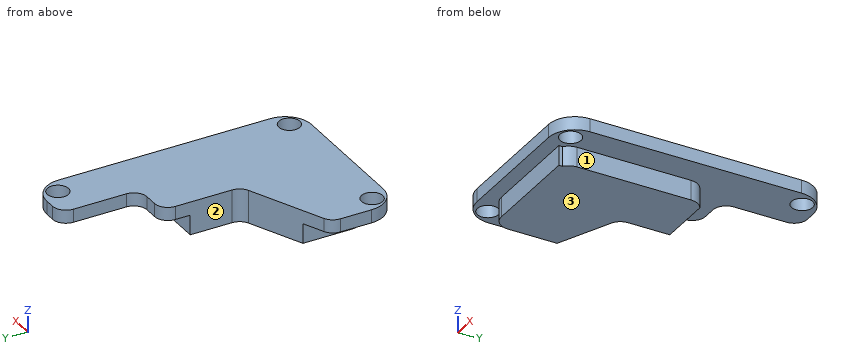
Autodesk Inventor part; units mm, degrees
ref_plane "YZ Plane" through (0, 0, 0) normal (1, 0, 0) x (0, 1, 0)
ref_plane "XZ Plane" through (0, 0, 0) normal (0, 1, 0) x (-1, 0, 0)
ref_plane "XY Plane" through (0, 0, 0) normal (0, 0, 1) x (1, 0, 0)
ref_plane "Arbeitsebene1" through (0, 0, 0) normal (0, 0, 1) x (1, 0, 0)
sketch "Skizze1" plane through (0, 0, 0) normal (0, 0, 1) x (1, 0, 0)
  line L0 (31.9586, -24.4) -> (31.9586, -21.8494)
  line L1 (31.9586, -24.4) -> (35.5793, -24.4)
  arc A0 (35.5793, -24.4) -> (36.5793, -23.4) centre (35.5793, -23.4) ccw
  line L2 (36.5793, -23.4) -> (36.5793, 14.6)
  arc A1 (36.5793, 14.6) -> (35.5793, 15.6) centre (35.5793, 14.6) ccw
  line L3 (35.5793, 15.6) -> (31.5586, 15.6)
  line L4 (31.5586, 15.6) -> (31.5586, -0.3724)
  arc A2 (32.766, -2.6793) -> (31.5586, -0.3724) centre (29.9586, -2.6793) ccw
  line L5 (32.766, -2.6793) -> (32.766, -19.8793)
  arc A3 (31.9586, -21.8494) -> (32.766, -19.8793) centre (29.9586, -19.8793) ccw
  line L6 (20.9586, -22.6867) -> (20.9586, -24.4)
  line L7 (20.9586, -22.6867) -> (16.1586, -22.6867)
  arc A4 (13.3512, -19.8793) -> (16.1586, -22.6867) centre (16.1586, -19.8793) ccw
  line L8 (13.3512, -19.8793) -> (13.3512, -2.6793)
  arc A5 (14.5586, -0.3724) -> (13.3512, -2.6793) centre (16.1586, -2.6793) ccw
  line L9 (14.5586, -0.3724) -> (14.5586, 15.6)
  line L10 (14.5586, 15.6) -> (10.5793, 15.6)
  arc A6 (10.5793, 15.6) -> (9.5793, 14.6) centre (10.5793, 14.6) ccw
  line L11 (9.5793, 14.6) -> (9.5793, -23.4)
  arc A7 (9.5793, -23.4) -> (10.5793, -24.4) centre (10.5793, -23.4) ccw
  line L12 (10.5793, -24.4) -> (20.9586, -24.4)
  circle A8 centre (12.0668, 4.4966) radius 1.4
  line L13 (31.5586, 15.6) -> (14.5586, 15.6)
  line L14 (31.9586, -24.4) -> (20.9586, -24.4)
  line L15 (10.5793, 15.6) -> (9.5793, 15.6)
  line L16 (9.5793, 15.6) -> (9.5793, 14.6)
  line L17 (35.5793, 15.6) -> (36.5793, 15.6)
  line L18 (36.5793, 15.6) -> (36.5793, 14.6)
  line L19 (9.5793, -23.4) -> (9.5793, -24.4)
  line L20 (9.5793, -24.4) -> (10.5793, -24.4)
  line L21 (35.5793, -24.4) -> (36.5793, -24.4)
  line L22 (36.5793, -24.4) -> (36.5793, -23.4)
extrude "Extrusion1" add sketch "Skizze1" along normal blind 2 contours L14 L6 L7 A4 L8 A5 L9 L13 L4 A2 L5 A3 L0 | L0 A3 L5 A2 L4 L3 A1 L2 A0 L1 | A0 L22 L21 | L12 A7 L11 A6 L10 L9 A5 L8 A4 L7 L6 | L20 L19 A7 | A1 L17 L18 | L16 L15 A6 | A8
ref_plane "Arbeitsebene2" through (0, 0, 0) normal (0, 0, 1) x (1, 0, 0)
sketch "Skizze2" plane through (0, 0, 2) normal (0, 0, 1) x (1, 0, 0)
  arc A0 (35.5793, -24.4) -> (36.5793, -23.4) centre (35.5793, -23.4) ccw
  line L0 (36.5793, -23.4) -> (36.5793, 14.6)
  arc A1 (36.5793, 14.6) -> (35.5793, 15.6) centre (35.5793, 14.6) ccw
  line L1 (35.5793, 15.6) -> (10.5793, 15.6)
  arc A2 (10.5793, 15.6) -> (9.5793, 14.6) centre (10.5793, 14.6) ccw
  line L2 (9.5793, 14.6) -> (9.5793, -23.4)
  arc A3 (9.5793, -23.4) -> (10.5793, -24.4) centre (10.5793, -23.4) ccw
  line L3 (10.5793, -24.4) -> (35.5793, -24.4)
  line L4 (34.0793, 13.1) -> (34.0793, -21.9)
  line L5 (34.0793, -21.9) -> (12.0793, -21.9)
  line L6 (12.0793, -21.9) -> (12.0793, 13.1)
  line L7 (12.0793, 13.1) -> (34.0793, 13.1)
  point P0 (8.0712, 15)
  point P1 (8.0712, -15)
  point P2 (38.0712, 15)
  point P3 (38.0712, -15)
  dimension "d21" = 2.5
hole "Bohrung1" at (34.0793, 13.1, 2) at (34.0793, -21.9, 2) at (12.0793, -21.9, 2) at (12.0793, 13.1, 2) direction (0, 0, -1) diameter 3.2 end through all
sketch "Skizze4" plane through (0, 0, 0) normal (0, 0, -1) x (-1, 0, 0)
  circle A0 centre (-34.0793, 13.1) radius 1.4
  circle A1 centre (-34.0793, -21.9) radius 1.4
  line L0 (-31.9586, -24.4) -> (-31.9586, -21.8494)
  line L1 (-31.9586, -24.4) -> (-35.5793, -24.4)
  arc A2 (-36.5793, -23.4) -> (-35.5793, -24.4) centre (-35.5793, -23.4) ccw
  line L2 (-36.5793, -23.4) -> (-36.5793, 14.6)
  arc A3 (-35.5793, 15.6) -> (-36.5793, 14.6) centre (-35.5793, 14.6) ccw
  line L3 (-35.5793, 15.6) -> (-31.5586, 15.6)
  line L4 (-31.5586, 15.6) -> (-31.5586, -0.3724)
  arc A4 (-31.5586, -0.3724) -> (-32.766, -2.6793) centre (-29.9586, -2.6793) ccw
  line L5 (-32.766, -2.6793) -> (-32.766, -19.8793)
  arc A5 (-32.766, -19.8793) -> (-31.9586, -21.8494) centre (-29.9586, -19.8793) ccw
  circle A6 centre (-12.0793, -21.9) radius 1.4
  circle A7 centre (-12.0793, 13.1) radius 1.4
  line L6 (-20.9586, -22.6867) -> (-20.9586, -24.4)
  line L7 (-20.9586, -22.6867) -> (-16.1586, -22.6867)
  arc A8 (-16.1586, -22.6867) -> (-13.3512, -19.8793) centre (-16.1586, -19.8793) ccw
  line L8 (-13.3512, -19.8793) -> (-13.3512, -2.6793)
  arc A9 (-13.3512, -2.6793) -> (-14.5586, -0.3724) centre (-16.1586, -2.6793) ccw
  line L9 (-14.5586, -0.3724) -> (-14.5586, 15.6)
  line L10 (-14.5586, 15.6) -> (-10.5793, 15.6)
  arc A10 (-9.5793, 14.6) -> (-10.5793, 15.6) centre (-10.5793, 14.6) ccw
  line L11 (-9.5793, 14.6) -> (-9.5793, -23.4)
  arc A11 (-10.5793, -24.4) -> (-9.5793, -23.4) centre (-10.5793, -23.4) ccw
  line L12 (-10.5793, -24.4) -> (-20.9586, -24.4)
  circle A12 centre (-12.0668, 4.4966) radius 1.4
  line L13 (-31.0586, -0.651) -> (-31.0586, 16.1)
  line L14 (-31.0586, 16.1) -> (-35.5793, 16.1)
  arc A13 (-35.5793, 16.1) -> (-37.0793, 14.6) centre (-35.5793, 14.6) ccw
  line L15 (-37.0793, 14.6) -> (-37.0793, -23.4)
  arc A14 (-37.0793, -23.4) -> (-35.5793, -24.9) centre (-35.5793, -23.4) ccw
  line L16 (-35.5793, -24.9) -> (-31.4586, -24.9)
  line L17 (-31.4586, -24.9) -> (-31.4586, -21.6326)
  arc A15 (-32.266, -19.8793) -> (-31.4586, -21.6326) centre (-29.9586, -19.8793) ccw
  line L18 (-32.266, -19.8793) -> (-32.266, -2.6793)
  arc A16 (-31.0586, -0.651) -> (-32.266, -2.6793) centre (-29.9586, -2.6793) ccw
  line L19 (-15.0586, 16.1) -> (-15.0586, -0.651)
  arc A17 (-13.8512, -2.6793) -> (-15.0586, -0.651) centre (-16.1586, -2.6793) ccw
  line L20 (-13.8512, -2.6793) -> (-13.8512, -19.8793)
  arc A18 (-16.1586, -22.1867) -> (-13.8512, -19.8793) centre (-16.1586, -19.8793) ccw
  line L21 (-16.1586, -22.1867) -> (-21.4586, -22.1867)
  line L22 (-21.4586, -24.4607) -> (-21.4586, -24.9)
  line L23 (-21.4586, -24.9) -> (-10.5793, -24.9)
  arc A19 (-10.5793, -24.9) -> (-9.0793, -23.4) centre (-10.5793, -23.4) ccw
  line L24 (-9.0793, -23.4) -> (-9.0793, 14.6)
  arc A20 (-9.0793, 14.6) -> (-10.5793, 16.1) centre (-10.5793, 14.6) ccw
  line L25 (-10.5793, 16.1) -> (-15.0586, 16.1)
  line L26 (-31.0586, 15.6607) -> (-15.0586, 15.6607)
  line L27 (-31.4586, -24.4607) -> (-21.4586, -24.4607)
  line L28 (-15.0586, -0.651) -> (-31.0586, -0.651)
  line L29 (-20.9586, -22.6867) -> (-20.9586, -22.1867)
  line L30 (-20.9586, -22.1867) -> (-31.9586, -22.1867)
  point P0 (0, 0)
  point P1 (-31.4586, -22.1867)
  dimension "d22" = 0.5
  dimension "d23" = 0.5
extrude "Extrusion2" add sketch "Skizze4" along normal blind 3 contours L28 A17 L20 A18 L21 L30 L17 A15 L18 A16
fillet "Rundung2" radius 4 4 edges at (9.5793, 15.6, 1) (36.5793, 15.6, 1) (9.5793, -24.4, 1) (36.5793, -24.4, 1)
sketch "Skizze5" plane through (0, 0, 0) normal (0, 0, -1) x (-1, 0, 0)
  circle A0 centre (-23.0793, -4.4) radius 4.25
  circle A1 centre (-12.0668, 4.4966) radius 1.4
  circle A2 centre (-34.0668, 4.4966) radius 1.4
  circle A3 centre (-12.0793, 13.1) radius 1.4
  circle A4 centre (-34.0793, -21.9) radius 1.4
  circle A5 centre (-34.0793, 13.1) radius 1.4
  circle A6 centre (-12.0793, -21.9) radius 1.4
  arc A7 (-29.0793, 13.6) -> (-31.0793, 15.6) centre (-31.0793, 13.6) ccw
  line L0 (-32.5793, 15.6) -> (-31.0793, 15.6)
  arc A8 (-32.5793, 15.6) -> (-36.5793, 11.6) centre (-32.5793, 11.6) ccw
  line L1 (-36.5793, -20.4) -> (-36.5793, 11.6)
  arc A9 (-36.5793, -20.4) -> (-32.5793, -24.4) centre (-32.5793, -20.4) ccw
  line L2 (-13.5793, -24.4) -> (-32.5793, -24.4)
  arc A10 (-13.5793, -24.4) -> (-9.5793, -20.4) centre (-13.5793, -20.4) ccw
  line L3 (-9.5793, 11.6) -> (-9.5793, -20.4)
  arc A11 (-9.5793, 11.6) -> (-13.5793, 15.6) centre (-13.5793, 11.6) ccw
  line L4 (-15.0793, 15.6) -> (-13.5793, 15.6)
  arc A12 (-15.0793, 15.6) -> (-17.0793, 13.6) centre (-15.0793, 13.6) ccw
  line L5 (-17.0793, 13.6) -> (-17.0793, 5.6)
  arc A13 (-19.0793, 3.6) -> (-17.0793, 5.6) centre (-19.0793, 5.6) ccw
  line L6 (-19.0793, 3.6) -> (-27.0793, 3.6)
  arc A14 (-29.0793, 5.6) -> (-27.0793, 3.6) centre (-27.0793, 5.6) ccw
  line L7 (-29.0793, 5.6) -> (-29.0793, 13.6)
  line L8 (-32.5793, 15.6) -> (-13.5793, 15.6)
  point P0 (0, 0)
extrude "Extrusion3" cut sketch "Skizze5" against normal blind 10 contours A7 L8 A12 L5 A13 L6 A14 L7
sketch "Skizze6" plane through (0, 0, 2) normal (0, 0, 1) x (1, 0, 0)
  line L0 (19.0793, 3.6) -> (27.0793, 3.6)
  line L1 (23.0793, 3.6) -> (23.0793, -8.2849)
  line L2 (23.0793, -8.2849) -> (9.5499, -14.3825)
  circle A0 centre (12.0793, 13.1) radius 1.6
  circle A1 centre (34.0793, -21.9) radius 1.6
  circle A2 centre (34.0793, 13.1) radius 1.6
  circle A3 centre (12.0793, -21.9) radius 1.6
  arc A4 (31.0793, 15.6) -> (29.0793, 13.6) centre (31.0793, 13.6) ccw
  line L3 (29.0793, 13.6) -> (29.0793, 5.6)
  arc A5 (27.0793, 3.6) -> (29.0793, 5.6) centre (27.0793, 5.6) ccw
  line L4 (27.0793, 3.6) -> (19.0793, 3.6)
  arc A6 (17.0793, 5.6) -> (19.0793, 3.6) centre (19.0793, 5.6) ccw
  line L5 (17.0793, 5.6) -> (17.0793, 13.6)
  arc A7 (17.0793, 13.6) -> (15.0793, 15.6) centre (15.0793, 13.6) ccw
  line L6 (15.0793, 15.6) -> (13.5793, 15.6)
  arc A8 (13.5793, 15.6) -> (9.5793, 11.6) centre (13.5793, 11.6) ccw
  line L7 (9.5793, 11.6) -> (9.5793, -20.4)
  arc A9 (9.5793, -20.4) -> (13.5793, -24.4) centre (13.5793, -20.4) ccw
  line L8 (13.5793, -24.4) -> (32.5793, -24.4)
  arc A10 (32.5793, -24.4) -> (36.5793, -20.4) centre (32.5793, -20.4) ccw
  line L9 (36.5793, -20.4) -> (36.5793, 11.6)
  arc A11 (36.5793, 11.6) -> (32.5793, 15.6) centre (32.5793, 11.6) ccw
  line L10 (32.5793, 15.6) -> (31.0793, 15.6)
  point P0 (0, 0)
  point P1 (9.5793, -14.3692)
extrude "Extrusion4" cut sketch "Skizze6" against normal blind 10 contours L0 L1 L2 L7 A8 L6 A7 L5 A6
fillet "Rundung3" radius 2 3 edges at (23.0793, 3.6, 1) (23.0793, -8.2849, -0.5) (9.5793, -14.3692, 1)
properties part number "00_ESP32_XIAO_Adapter_lid_a4988"
Can you work these out from the model? Positions are in its coordinate system, mm. Face numbers are marked on the shaded views. A direction names the side the tool comes from. Coordinates: 2 decimals unless noted, no trailing zeros. Write each loop counter-clockwise with the first axis right and the second up, starting at its lowest first coordinate (ties: lowest second). Pieces come first, ordered by that corner, then holes. Notation, with made-up numbers: (-20.75, 80) -> (-12.75, 80) arc R5 cw to (-12.75, 87) -> close; hole circle Ø4 at (45.25, 22.5). An arc over 180 degrees is marked (long way). Write each question's results on one line, items separated by ' | '. Start each with the question number.
Q1. Imagine slicing it at D-D (z = 1.55). Write out the boundary of the cut face in (x, y), then the cut area to 3 significant figures.
Q2. On a 3-axis mill with a long thin cutter (end or side, diameter ignored), from which of +Z, -Z, +X, -X, +Y, -Y can I reach the whole of each face in a straight line? I mean the marked faces 1, 2 and 3. Say none if no direction works.
Q3. If I drill on probe 1 along X at (y, z) = (-21.9, 1.1); probe 2 along X at (y, z) = (13.1, 0.7); probe 3 along Y at (x, z) = (25.5, -1.6), over which ranges is the centre line in solid material (lowest first)?
Q4. I'm going to push flat-ended pins straight in: pin 1 (0.6 mm diameter, centred on y = -22, z = -2, fed in from +X); pin 2 (1 mm diameter, centred on x = 31, z = -1.5, fed in from +Y); pin 3 (1.5 mm diameter, centred on y = -15.5, z = -1.5, fed in from -X); pin 4 (2 mm diameter, centred on x = 20.5, y = -2, fed in from +Z). Where does each tip first touch, or does it pass through?
Q5. Imagine slicing it at A-A (z = -1.4). Write out the boundary of the cut face in (x, y).
Q6. Imagine slicing it at C-C (y = 13.1). Write out the boundary of the cut face in (x, z).
Q7. Imagine slicing it at B-B (x = 35.25). Write out the boundary of the cut face in (y, z).
Taken from the geometry:
1) outline: (9.58, -20.4) arc R4 ccw to (13.58, -24.4) -> (32.58, -24.4) arc R4 ccw to (36.58, -20.4) -> (36.58, 11.6) arc R4 ccw to (32.58, 15.6) -> (31.08, 15.6) arc R2 ccw to (29.08, 13.6) -> (29.08, 5.6) arc R2 cw to (27.08, 3.6) -> (25.08, 3.6) arc R2 ccw to (23.08, 1.6) -> (23.08, -6.99) arc R2 cw to (21.9, -8.82) -> (10.76, -13.84) arc R2 ccw to (9.58, -15.66) -> close; hole circle Ø3.2 at (12.08, -21.9); hole circle Ø3.2 at (34.08, -21.9); hole circle Ø3.2 at (34.08, 13.1) | area: 609 mm^2
2) face 1: -Z, +X, +Y, -Y | face 2: +Z, -Z, -X, +Y | face 3: -Z, +X, -X, +Y, -Y
3) probe 1: x = 9.87 to 10.48, 13.68 to 32.48, 35.68 to 36.29 | probe 2: x = 29.08 to 32.48, 35.68 to 36.29 | probe 3: y = -22.19 to -0.65
4) pin 1: stops at x = 31.46 | pin 2: stops at y = -0.65 | pin 3: stops at x = 13.85 | pin 4: passes through
5) outline: (13.85, -19.88) arc R2.31 ccw to (16.16, -22.19) -> (31.46, -22.19) -> (31.46, -21.63) arc R2.31 ccw to (32.27, -19.88) -> (32.27, -2.68) arc R2.31 ccw to (31.06, -0.65) -> (23.08, -0.65) -> (23.08, -6.99) arc R2 cw to (21.9, -8.82) -> (13.85, -12.44) -> close
6) outline: (29.08, 0) -> (32.48, 0) -> (32.48, 2) -> (29.08, 2) -> close; (35.68, 0) -> (36.29, 0) -> (36.29, 2) -> (35.68, 2) -> close
7) outline: (-23.38, 0) -> (-22.99, 0) -> (-22.99, 2) -> (-23.38, 2) -> close; (-20.81, 0) -> (12.01, 0) -> (12.01, 2) -> (-20.81, 2) -> close; (14.19, 0) -> (14.58, 0) -> (14.58, 2) -> (14.19, 2) -> close
